Model file for the job. Use its own axes, mm. A direction names the side the tool comes from. Round coordinates to 2 decimals unless told otherwise and drop trailing zeros. Order: outer loops, then holes, each group sorted by start corner. A loop starts at its lowest first (then second) coordinate and runs counter-clockwise, first axis right, second up. Notation, with made-up numbers: (65.5, 4) - (92.5, 4) arc R23 ccw to (92.5, 17) - close; hole circle Ø9 at (42.25, 36). An arc over 180 degrees is marked (long way). Answer as CSV lines item,"result". Start each with the question number.
1. Band-saw the part on C-C on y = 14.5. List the corners of the cut face in (x, z), then the cut area to 3 significant figures.
2. Pin check, flat tips, straight feed: pin 1 Ø4 at (x, y) = (1.5, 39) entering from -Z; pin 2 Ø2 at (x, z) = (0, -1) entering from +Y; pin 3 Ø3 at (x, y) = (1.5, 44) entering from +Z; pin 4 Ø2 at (y, z) = (56, -0.5) entering from -X. Stop position of each tip, or through.
3. Band-saw the part on D-D on x = 3. List the corners of the cut face in (y, z), then the cut area to 3 significant figures.
4. Pull direction Z, two halves, no side cores. Call faces 4 (the face through (-1.098, 56.014, 1.866)), 5 (the face through (-3.417, 55.479, -0.759)), 6 (the face through (-0.7, 57, 2.3)): released by +Z, released by -Z, zero draft, split by the parting line, or undercut.
5. Band-saw the part on A-A on z = 0. List the corners of the cut face in (x, y).
6. 3-axis set-ups, long thin cutter, end or side, ignore diameter. For faces 1 (the face through (-2.44, 26.62, -0.54)), 2 (the face through (-2.165, 56, 0)), 3 (the face through (0, 0, 0)): which of +Z, -Z, +X, -X, +Y, -Y reach the whole face in a straight line?
7. Wall check: line 1 along Z through (x, y) = (1.25, 15); line 2 along Y through (x, z) = (2.5, 1); line 3 along Y through (x, z) = (0, -1.25). Give the ranges that are in metal, low to high. Write a range as [from, to].
8. Band-saw the part on B-B on x = 0.5. List the corners of the cut face in (y, z), then the cut area to 3 significant figures.
```python
from build123d import *

# Parameters (mm, degrees)
SKETCH1_R          = 2.5
SCREW_LENGTH_DEPTH = 54
SKETCH2_R          = 3.5
SCREW_CAP_DEPTH    = 3
SCREW_HOLE_DEPTH   = 2


with BuildPart() as part:
    # Sketch1 → Screw Length (new body)
    with BuildSketch(Plane(origin=(0, 0, 0), x_dir=(1, 0, 0), z_dir=(0, 1, 0))):
        with Locations(Location((0, 0, 0), (0, 0, 270))):
            Circle(SKETCH1_R)
    extrude(amount=SCREW_LENGTH_DEPTH)

    # Sketch2 → Screw Cap (add)
    with BuildSketch(Plane(origin=(0, 54, 0), x_dir=(1, 0, 0), z_dir=(0, 1, 0))):
        with Locations(Location((0, 0, 0), (0, 0, 270))):
            Circle(SKETCH2_R)
    extrude(amount=SCREW_CAP_DEPTH)

    # Sketch3 → Screw Hole (cut)
    with BuildSketch(Plane(origin=(0, 57, 0), x_dir=(1, 0, 0), z_dir=(0, 1, 0))):
        Polygon((0, 2.5), (-2.165063509, 1.25), (-2.165063509, -1.25), (0, -2.5), (2.165063509, -1.25), (2.165063509, 1.25), align=None)
    extrude(amount=-SCREW_HOLE_DEPTH, mode=Mode.SUBTRACT)


solid = part.part
```
Reply:
1,outline,"circle Ø5 at (0, 0)"
1,area,"19.6 mm2"
2,pin 1,"stops at z = -2.5"
2,pin 2,"stops at y = 55"
2,pin 3,"stops at z = 2.5"
2,pin 4,"stops at x = -3.5"
3,outline,"(54, -1.8) - (57, -1.8) - (57, 1.8) - (54, 1.8) - close"
3,area,"10.8 mm2"
4,face 4,"undercut"
4,face 5,"split by the parting line"
4,face 6,"zero draft"
5,outline,"(-3.5, 54) - (-2.5, 54) - (-2.5, 0) - (2.5, 0) - (2.5, 54) - (3.5, 54) - (3.5, 57) - (2.17, 57) - (2.17, 55) - (-2.17, 55) - (-2.17, 57) - (-3.5, 57) - close"
6,face 1,"-Y"
6,face 2,"+Y"
6,face 3,"+Z, -Z, +X, -X, -Y"
7,line 1,"z = [-2.17, 2.17]"
7,line 2,"y = [54, 57]"
7,line 3,"y = [0, 55]"
8,outline,"(0, -2.45) - (54, -2.45) - (54, -3.46) - (57, -3.46) - (57, -2.21) - (55, -2.21) - (55, 2.21) - (57, 2.21) - (57, 3.46) - (54, 3.46) - (54, 2.45) - (0, 2.45) - close"
8,area,"276 mm2"
